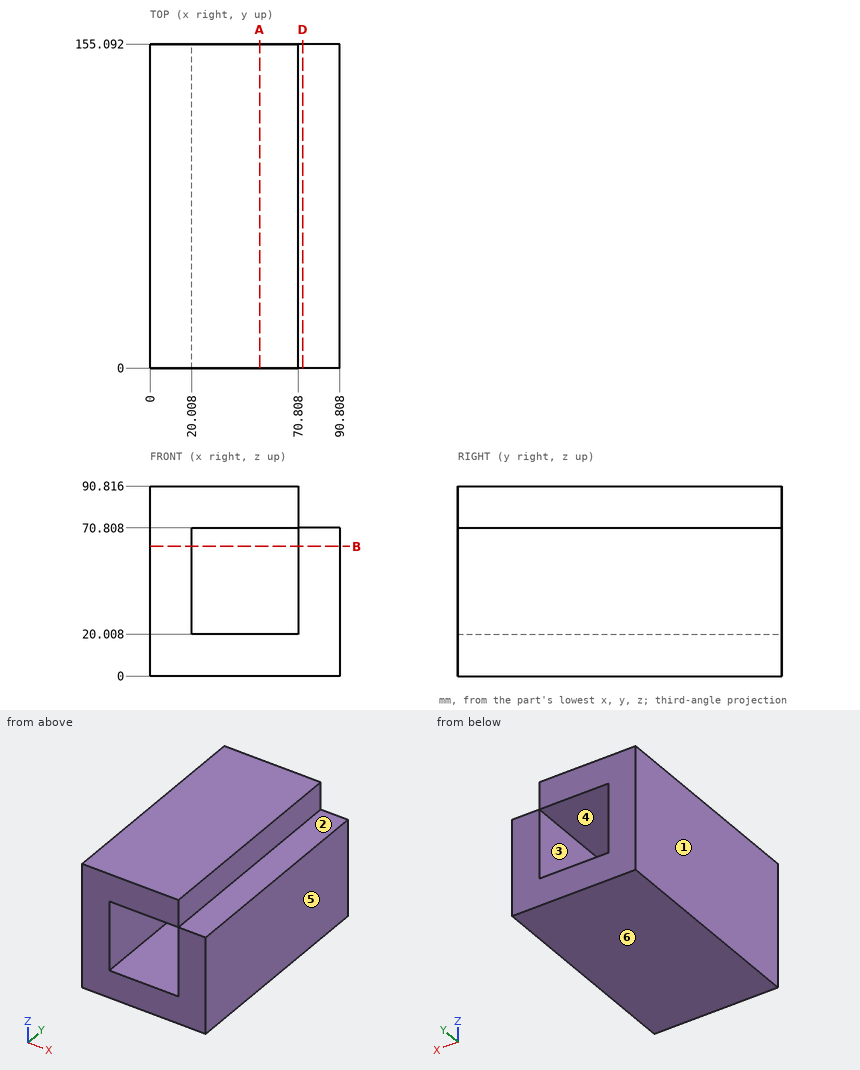
Answer from the drawing. Dimensions are ordinates in mm from the lowest x, y and z of the part. A direction names the side the tool comes from. Round coordinates to 2 decimals unless told otherwise and drop trailing zeros. Loops run counter-clockwise (first coordinate to the right, second up) from the corner with the lowest first, then second, coordinate; pieces in that order, holes last.
1) A cutting plane is placed at D-D on x = 73. Determine the outline of the cut face in (y, z), plus the area to 3 significant figures.
Outcome:
outline: (0, 0) - (155.09, 0) - (155.09, 70.81) - (0, 70.81) - close
area: 11,000 mm2
2) Given P1, Ø10, axis at y = 81, z = 81, coming from the +X side, flat-ended and moving along its own axis, determine where the tip first touches the part or whether it passes through.
Outcome:
P1: stops at x = 70.81
3) A cutting plane is placed at B-B on z = 62. Determine the outline of the cut face in (x, y).
Outcome:
outline: (0, 0) - (20.01, 0) - (20.01, 155.09) - (0, 155.09) - close; (70.81, 0) - (90.81, 0) - (90.81, 155.09) - (70.81, 155.09) - close
4) For the marked faces 1, 2 and 3, determine the directions among +Z, -Z, +X, -X, +Y, -Y from which every point of the face is accessible in a straight line to the end or side of a thin tool.
Outcome:
face 1: +Z, -Z, -X, +Y, -Y
face 2: +Z, +X, +Y, -Y
face 3: +Y, -Y
5) Consider line 1 (Z direction, x = 22, y = 26.5); line 2 (X direction, y = 64, z = 70); line 3 (X direction, y = 115, z = 81). Determine where each line is inside the solid, lowest interval first.
Outcome:
line 1: z = 0 to 20.01, 70.81 to 90.82
line 2: x = 0 to 20.01, 70.81 to 90.81
line 3: x = 0 to 70.81
6) For a pull along Z with two mould halves and no side action, classify the marked faces 4, 5 and 6 as released by +Z, released by -Z, zero draft, split by the parting line, or undercut.
Outcome:
face 4: undercut
face 5: zero draft
face 6: released by -Z
7) A cutting plane is placed at A-A on x = 52.5. Determine the outline of the cut face in (y, z), plus the area to 3 significant figures.
Outcome:
outline: (0, 0) - (155.09, 0) - (155.09, 20.01) - (0, 20.01) - close; (0, 70.81) - (155.09, 70.81) - (155.09, 90.82) - (0, 90.82) - close
area: 6,210 mm2
